Here's the drawing with two shaded views (mm, measured from the low corner). I have some questions. A direction names the side the tool comes from. Round coordinates to 2 decimals unless told otherwise and drop trailing zeros. Loops run counter-clockwise (first coordinate to the right, second up) from the corner with the lowest first, then second, coordinate; pieces in that order, holes last. Notation, with made-up numbers: (35.25, 4.5) -> (54.25, 4.5) arc R19 cw to (54.25, 20.5) -> close; hole circle Ø11 at (-3, 2). An arc over 180 degrees is marked (long way). One line per item, written item: value. Start each with the question number.
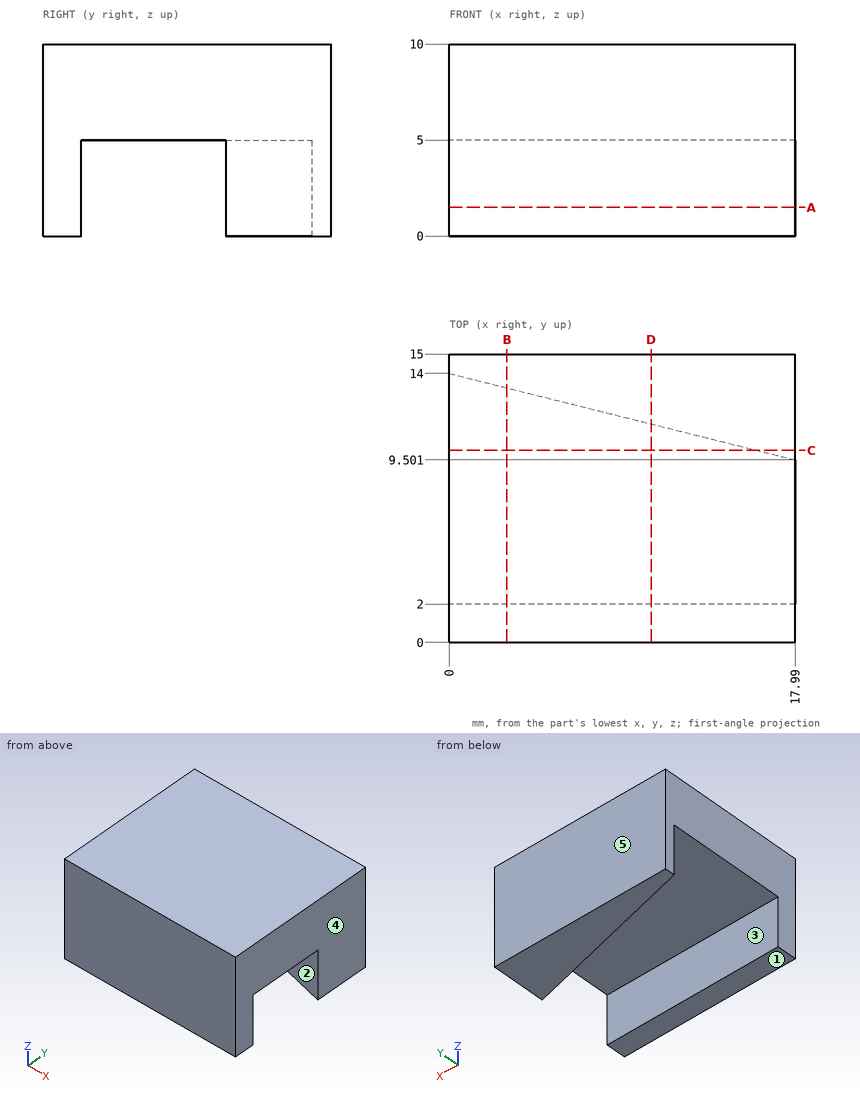
Q1. If I drill on line 1 along Z through (x, y) = (6.5, 10); line 2 along Y through (x, z) = (9, 1.75); line 3 along Y through (x, z) = (5, 3.5), over which ranges is the centre line in solid material (lowest first)?
Q2. I want a section at B-B on x = 3. Please give me the cut outline in (y, z).
Q3. If we mould it in two halves opening along Y, with no side actions, what happens to the marked faces 3, 4 and 5? For each: released by +Y, released by -Y, zero draft, split by the parting line, or undercut.
Q4. I want a section at D-D on x = 10.5. Please give me the cut outline in (y, z).
Q5. Which directions (+Z, -Z, +X, -X, +Y, -Y) give clear straight access to the entire face, cutting with the end or side of a thin tool? Please do the marked faces 1 and 2.
Q6. I want a section at A-A on z = 1.5. Please give me the cut outline in (x, y).
Q7. Will this pin go through, and if not, where does the flat tip stop? P1, Ø6, axis at x = 11, y = 6.5, coming from the -Z side.
Q8. I want a section at C-C on y = 10. Please give me the cut outline in (x, z).
Answers below:
1. line 1: z = 5 to 10
1. line 2: y = 0 to 2, 11.75 to 15
1. line 3: y = 0 to 2, 12.75 to 15
2. outline: (0, 0) -> (2, 0) -> (2, 5) -> (13.25, 5) -> (13.25, 0) -> (15, 0) -> (15, 10) -> (0, 10) -> close
3. face 3: undercut
3. face 4: zero draft
3. face 5: released by +Y
4. outline: (0, 0) -> (2, 0) -> (2, 5) -> (11.37, 5) -> (11.37, 0) -> (15, 0) -> (15, 10) -> (0, 10) -> close
5. face 1: -Z, +X, -X, +Y, -Y
5. face 2: -Z, -X
6. outline: (0, 0) -> (17.99, 0) -> (17.99, 2) -> (0, 2) -> close; (0, 14) -> (17.99, 9.5) -> (17.99, 15) -> (0, 15) -> close
7. P1: stops at z = 5
8. outline: (0, 5) -> (16, 5) -> (16, 0) -> (17.99, 0) -> (17.99, 10) -> (0, 10) -> close
